Source: CAD feature listing. Evaluate the final solid. Frame: model axes, mm. Round coordinates to 2 decimals unless told otherwise and drop trailing zeros. Write each loop counter-clockwise with the first axis right and the second up, starting at its lowest first coordinate (ties: lowest second). Pieces come first, ordered by that corner, then holes. Notation, with made-up numbers: M 23,32.5 L 61,32.5 A21 ccw 61,57.5 Z; hole C 39,19.5 d5. An arc over 180 degrees is marked long. Answer in a Markdown table with one row per item. Add a question column.
Item 1: Material intervals for probe 1 along Z at (x, y) = (-45.5, 10); probe 2 along Z at (x, y) = (-44, -17); probe 3 along X at (y, z) = (-29, 39.5), sorted ascending.
Item 2: Cut plane A-A on y = 12.5. Return loops of the section in (x, z), and give its area (3 significant figures).
Item 3: Cut plane B-B on x = -32. Return loops of the section in (y, z), and give its area (3 significant figures).
Item 4: Contact query for flat-ended pins moving along their axis: pin 1 (1 mm diameter, centred on x = 22, y = -7, fed in from +Z); pin 2 (2 mm diameter, centred on y = 1, z = 19.5, fed in from -X); pin 3 (5 mm diameter, centred on y = -18, z = 18, fed in from -X). Output: stop coordinate, or through.
from build123d import *

# Parameters (mm, degrees)
F0_W        = 128.2073557377
F0_H        = 88.262155652
F1_DEPTH    = 50.68946
F2_T1_DEPTH = 361.3524449255
F3_T1_DEPTH = 361.352454187


# Not quite as in the source:
# - a fillet or chamfer that OpenCascade refuses, or shapes differently, is made with other operations: its cross-section is extruded or revolved along the edge and cut away or added


with BuildPart() as f1:
    # F0 (on Top) → F1 (new body)
    with BuildSketch(Plane.XY):
        Rectangle(F0_W, F0_H)
    extrude(amount=F1_DEPTH)

    # F2: fillet of radius 54.7702974041 on 1 edges, made by hand

    # F2_s2 → F2_t1 (cut)
    with BuildSketch(Plane.XZ.offset(-180.6762224627)):
        with BuildLine():
            ThreePointArc((-64.1036778688, 0), (-46.7433494099, 36.0644870809), (-9.4856200142, 50.68946))
            Line((-9.4856200142, 50.68946), (-64.1036778688, 50.68946))
            Line((-64.1036778688, 50.68946), (-64.1036778688, 0))
        make_face()
    extrude(amount=F2_T1_DEPTH, mode=Mode.SUBTRACT)

    # F3: fillet of radius 54.7702994 on 1 edges, made by hand

    # F3_s2 → F3_t1 (cut)
    with BuildSketch(Plane.XZ.offset(-180.6762270935)):
        with BuildLine():
            ThreePointArc((64.1036778688, 0), (46.7433482365, 36.064487178), (9.4856181618, 50.68946))
            Line((9.4856181618, 50.68946), (64.1036778688, 50.68946))
            Line((64.1036778688, 50.68946), (64.1036778688, 0))
        make_face()
    extrude(amount=F3_T1_DEPTH, mode=Mode.SUBTRACT)


solid = f1.part
Results below:
| question | item | result |
|---|---|---|
| 1 | probe 1 | 0 to 37.18 |
| 1 | probe 2 | 0 to 38.45 |
| 1 | probe 3 | -42.66 to 42.66 |
| 2 | outline | M -64.1,0 L 64.1,0 A54.77 ccw 9.49,50.69 L -9.49,50.69 A54.77 ccw Z |
| 2 | area | 5,230 mm2 |
| 3 | outline | M -44.13,0 L 44.13,0 L 44.13,45.85 L -44.13,45.85 Z |
| 3 | area | 4,050 mm2 |
| 4 | pin 1 | z = 49.36 |
| 4 | pin 2 | x = -59.38 |
| 4 | pin 3 | x = -60.64 |
